from build123d import *

# Parameters (mm, degrees)
SKETCH1_W           = 23.99999232
SKETCH1_H           = 16.699994656
BOSS_EXTRUDE1_DEPTH = 6


with BuildPart() as part:
    # Sketch1 → Boss-Extrude1 (new body)
    with BuildSketch(Plane.XY):
        with Locations((252.776898883, 87.516141094)):
            Rectangle(SKETCH1_W, SKETCH1_H)
        Polygon((254.420508276, 82.46614271), (254.600328979, 82.90026829), (254.661662472, 83.366142422), (254.600328979, 83.832016554), (254.420508276, 84.266142134), (254.134454846, 84.638934221), (253.76166276, 84.92498765), (253.32753718, 85.104808353), (252.861663048, 85.166141846), (252.395788915, 85.104808353), (251.961663336, 84.92498765), (251.588871249, 84.638934221), (251.30281782, 84.266142134), (251.122997117, 83.832016554), (251.061663624, 83.366142422), (251.122997117, 82.90026829), (251.30281782, 82.46614271), (251.588871249, 82.093350624), (251.961663336, 81.807297194), (252.395788915, 81.627476491), (252.861663048, 81.566142998), (253.32753718, 81.627476491), (253.76166276, 81.807297194), (254.134454846, 82.093350624), align=None, mode=Mode.SUBTRACT)
        Polygon((260.30990578, 88.127474411), (260.775779912, 88.066140918), (261.241654045, 88.127474411), (261.675779624, 88.307295114), (262.048571711, 88.593348544), (262.33462514, 88.96614063), (262.514445843, 89.40026621), (262.575779336, 89.866140342), (262.514445843, 90.332014474), (262.33462514, 90.766140054), (262.048571711, 91.138932141), (261.675779624, 91.42498557), (261.241654045, 91.604806273), (260.775779912, 91.666139766), (260.30990578, 91.604806273), (259.8757802, 91.42498557), (259.502988114, 91.138932141), (259.216934685, 90.766140054), (259.037113982, 90.332014474), (258.975780488, 89.866140342), (259.037113982, 89.40026621), (259.216934685, 88.96614063), (259.502988114, 88.593348544), (259.8757802, 88.307295114), align=None, mode=Mode.SUBTRACT)
        Polygon((246.335746671, 90.766140054), (246.049693242, 91.138932141), (245.676901155, 91.42498557), (245.242775575, 91.604806273), (244.776901443, 91.666139766), (244.311027311, 91.604806273), (243.876901731, 91.42498557), (243.504109644, 91.138932141), (243.218056215, 90.766140054), (243.038235512, 90.332014474), (242.976902019, 89.866140342), (243.038235512, 89.40026621), (243.218056215, 88.96614063), (243.504109644, 88.593348544), (243.876901731, 88.307295114), (244.311027311, 88.127474411), (244.776901443, 88.066140918), (245.242775575, 88.127474411), (245.676901155, 88.307295114), (246.049693242, 88.593348544), (246.335746671, 88.96614063), (246.515567374, 89.40026621), (246.576900867, 89.866140342), (246.515567374, 90.332014474), align=None, mode=Mode.SUBTRACT)
        Polygon((251.594211482, 88.030941424), (251.614308424, 87.934752995), (251.674599249, 87.845978104), (251.91576255, 87.690668939), (252.277126402, 87.585307372), (252.718115827, 87.55018685), (253.159105252, 87.585307372), (253.520469104, 87.690668939), (253.761632405, 87.845978104), (253.82192323, 87.934752995), (253.842020171, 88.030941424), (253.842020171, 91.377359106), (253.82192323, 91.473547535), (253.761632405, 91.562322426), (253.520469104, 91.717631591), (253.159105252, 91.822993158), (252.718115827, 91.85811368), (252.277126402, 91.822993158), (251.91576255, 91.717631591), (251.674599249, 91.562322426), (251.614308424, 91.473547535), (251.594211482, 91.377359106), align=None, mode=Mode.SUBTRACT)
    extrude(amount=BOSS_EXTRUDE1_DEPTH)


solid = part.part
CAD build for the part. Positions are in the model's coordinates, mm. Round coordinates to 2 decimals unless told otherwise and drop trailing zeros. Answer as a JSON object with one key per item and string values.
(1) Probe probe 1 along X at (y, z) = (88, 1.15); probe 2 along X at (y, z) = (89.75, 2.9); probe 3 along X at (y, z) = (89, 2.35). List the from-to ranges inside material, lowest first. Write a range as [from, to].
Reported:
{"probe 1": "x = [240.78, 251.6], [253.84, 264.78]", "probe 2": "x = [240.78, 242.99], [246.56, 251.59], [253.84, 258.99], [262.56, 264.78]", "probe 3": "x = [240.78, 243.2], [246.35, 251.59], [253.84, 259.2], [262.35, 264.78]"}
(2) Band-saw the part on A-A, the plane z = 0.7. Count the separate pieces of the cut face and the enclosed holes in it, then the cut area to 3 significant figures.
Reported:
{"separate pieces": "1", "enclosed holes": "4", "area": "361 mm^2"}
(3) Two-plate mould, pull along Y, no slides. Class faces 1 (the face through (253, 79.166, 3)), 2 (the face through (251.594, 90, 3)), 3 (the face through (240.777, 87, 3)), 4 (the face through (253.842, 90, 3)): +Y half, -Y half, draft (parallel to the pull), parting line (faces both ways), or undercut.
Reported:
{"face 1": "-Y half", "face 2": "undercut", "face 3": "draft", "face 4": "undercut"}
